Geometry: final body of the model. Coordinates: model frame, mm. A direction names the side the tool comes from. Coordinates: 2 decimals unless noted, no trailing zeros. Loops run counter-clockwise (first coordinate to the right, second up) from the corner with the lowest first, then second, coordinate; pieces in that order, holes last. Notation, with made-up numbers: (-18, 16.5) - (37, 16.5) arc R26 cw to (37, 44.5) - close; hole circle Ø10 at (69.25, 46). An arc over 180 degrees is marked (long way). Return JSON: item names as keys, results as strings.
Autodesk Inventor part; units mm, degrees
ref_plane "YZ Plane" through (0, 0, 0) normal (1, 0, 0) x (0, 1, 0)
ref_plane "XZ Plane" through (0, 0, 0) normal (0, 1, 0) x (-1, 0, 0)
ref_plane "XY Plane" through (0, 0, 0) normal (0, 0, 1) x (1, 0, 0)
sketch "Sketch1" plane through (0, 0, 0) normal (0, 0, 1) x (1, 0, 0)
  line L0 (0, 0) -> (25.4, 0)
  line L1 (25.4, 0) -> (25.4, 25.4)
  line L2 (25.4, 25.4) -> (0, 25.4)
  line L3 (0, 25.4) -> (0, 0)
  line L4 (1.5875, 23.8125) -> (23.8125, 23.8125)
  line L5 (23.8125, 23.8125) -> (23.8125, 1.5875)
  line L6 (23.8125, 1.5875) -> (1.5875, 1.5875)
  line L7 (1.5875, 1.5875) -> (1.5875, 23.8125)
  dimension "d0" = 25.4
  dimension "d2" = 25.4
  dimension "d3" = 1.5875
extrude "Extrusion1" add sketch "Sketch1" along normal blind 495.3
sketch "Sketch2" plane through (0, 25.4, 0) normal (0, 1, 0) x (1, 0, 0)
  line L0 (25.4, 0) -> (0, 0)
  line L1 (0, 0) -> (0, -495.3)
  line L2 (25.4, -495.3) -> (0, -495.3)
  line L3 (25.4, 0) -> (25.4, -495.3)
  line L4 (25.4, -495.3) -> (0, -469.9)
  line L5 (25.4, 0) -> (0, -25.4)
  dimension "d6" = 135
  dimension "d7" = 45
extrude "Extrusion2" cut sketch "Sketch2" against normal blind 495.3 contours L5 L1 L0 | L2 L1 L4
sketch "Sketch3" plane through (25.4, 0, 0) normal (0, -1, 0) x (1, 0, 0)
  circle A0 centre (-12.7, 69.85) radius 3.3782
  circle A1 centre (-12.7, 47.625) radius 3.3782
  circle A2 centre (-12.7, 425.45) radius 3.3782
  circle A3 centre (-12.7, 447.675) radius 3.3782
  circle A4 centre (-12.7, 266.7) radius 3.3782
  line L0 (-23.1775, 257.9688) -> (-23.1775, 275.4313)
  line L1 (-6.35, 257.9688) -> (-23.1775, 257.9688)
  line L2 (-6.35, 275.4313) -> (-6.35, 257.9688)
  line L3 (-6.35, 275.4313) -> (-23.1775, 275.4313)
  point P0 (-25.4, 0)
extrude "Extrusion3" cut sketch "Sketch3" against normal blind 25.4 contours A0 | A1 | A2 | A3 | A4
sketch "Sketch4" plane through (0, 0, 25.4) normal (-1, 0, 0) x (0, 0, 1)
  circle A0 centre (431.8, 12.7) radius 3.3782
  circle A1 centre (381, 12.7) radius 3.3782
  circle A2 centre (12.7, 12.7) radius 3.3782
  circle A3 centre (63.5, 12.7) radius 3.3782
  point P0 (-25.4, 0)
extrude "Extrusion4" cut sketch "Sketch4" against normal blind 25.4
properties part number "Rebuild Shooter Tower Top Tube 2" material "Aluminum 6061"
Item 1: Mould query, pull axis X, two halves, no side actions, for faces 1 (the face through (12.8, 24, 482.7)), 2 (the face through (13, 1.588, 244)), 3 (the face through (25.4, 13, 244)), 4 (the face through (13, 0, 244)). Classes: +X half, -X half, draft (parallel to the pull), parting line (faces both ways), or undercut.
Worked out:
{"face 1": "-X half", "face 2": "undercut", "face 3": "+X half", "face 4": "draft"}
Item 2: Reachability of faces 5 (the face through (23.812, 13, 244)), 6 (the face through (13, 25.4, 244)) from +Z, -Z, +X, -X, +Y, -Y: full face, straight path, thin tool, end or side. Return the list, or none.
Worked out:
{"face 5": "+Z, -Z", "face 6": "+Z, -Z, +X, -X, +Y"}
Item 3: Section query B-B, the plane y = 5.5. Return loops of the section in (x, z).
Worked out:
{"outline": "(0, 25.4) - (1.59, 23.81) - (1.59, 471.49) - (0, 469.9) - close; (23.81, 1.59) - (25.4, 0) - (25.4, 495.3) - (23.81, 493.71) - close"}
Item 4: Ray query, probe 1 along X at (y, z) = (14.75, 217); probe 2 along X at (y, z) = (1.15, 425.45). Return the intervals inside material, ascending. Write a range as from..to.
Worked out:
{"probe 1": "0..1.59, 23.81..25.4", "probe 2": "0..9.32, 16.08..25.4"}
Item 5: Section query A-A, the plane z = 104. Return loops of the section in (x, y), and give its area (3 significant figures).
Worked out:
{"outline": "(0, 0) - (25.4, 0) - (25.4, 25.4) - (0, 25.4) - close; hole (1.59, 1.59) - (23.81, 1.59) - (23.81, 23.81) - (1.59, 23.81) - close", "area": "151 mm^2"}
Item 6: First-contact query: pin 1 Ø9 at (y, z) = (12.7, 88.9) entering from -X; pin 2 Ø1.5 at (x, y) = (3.5, 19) entering from +Z; pin 3 Ø6 at (x, y) = (2.5, 22) entering from +Z; pin 4 Ø12 at (x, y) = (19.5, 11) entering from -Z. Flat tips, straight axial feed; report the tip coordinate or a pass-through.
Worked out:
{"pin 1": "x = 0", "pin 2": "through", "pin 3": "z = 474.79", "pin 4": "z = 0"}
